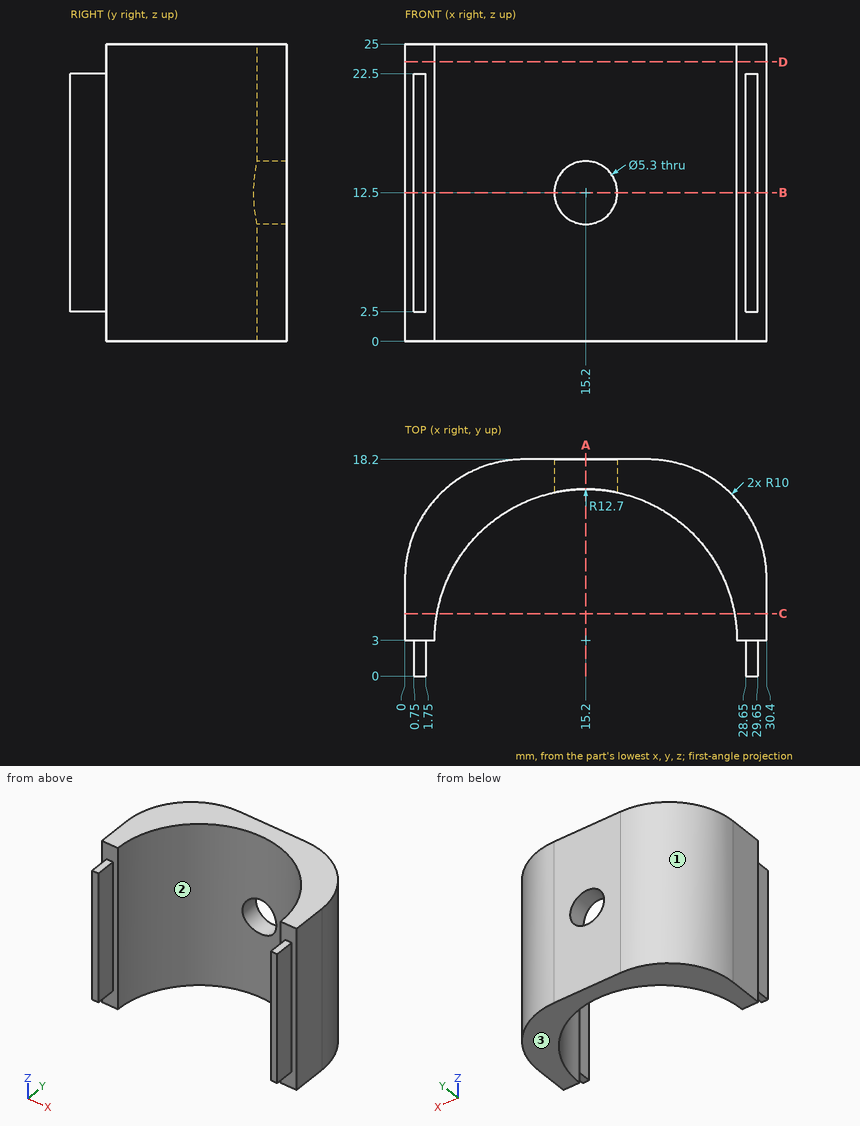
Geometry: see drawing. Coordinates: mm, zero at the bounding-box minimum. Coordinates: 2 decimals unless noted, no trailing zeros. Write each loop counter-clockwise with the first axis right and the second up, starting at its lowest first coordinate (ties: lowest second). Pieces come first, ordered by that corner, then holes. Notation, with made-up numbers: (-37, -19) - (-2, -19) arc R16 cw to (-2, -1) - close; hole circle Ø10 at (-18.5, -38.75). An arc over 180 degrees is marked (long way). Put each result on its own line as item: value. Start each with the question number.
1) Contact query for flat-ended pins moving along their axis: pin 1 (6 mm diameter, centred on x = 15.2, z = 12.5, fed in from -Y); pin 2 (3 mm diameter, centred on x = 1, z = 11.5, fed in from -Y); pin 3 (4 mm diameter, centred on y = 13, z = 18.5, fed in from +X); pin 4 (2.5 mm diameter, centred on y = 1, z = 8, fed in from -X). Output: stop coordinate, or through.
2) Cut plane B-B (z = 12.5). Return the cut outline in (x, y).
3) Ray query, L1, parallel to Z at x = 15.2, y = 16.65; L2, parallel to X at y = 2.5, z = 22; L3, parallel to X at y = 11.5, z = 10.75. Return the intervals inside material, ascending.
4) Cut plane C-C (y = 5.25). Return the cut outline in (x, z), plus the area to 3 significant figures.
5) Mould query, pull axis X, two halves, no side actions, for the marked faces 1, 2 and 3. Classes: pulls with the +X half, pulls with the -X half, needs draft (parallel to the pull), parting line crosses it, or undercut.
6) Cut plane D-D (z = 23.5). Return the cut outline in (x, y), plus the area to 3 significant figures.
7) Cut plane A-A (x = 15.2). Return the cut outline in (y, z), plus the area to 4 significant figures.
Resolved:
1. pin 1: stops at y = 15.34
1. pin 2: stops at y = 0
1. pin 3: stops at x = 30
1. pin 4: stops at x = 0.75
2. outline: (0, 3) - (0.75, 3) - (0.75, 0) - (1.75, 0) - (1.75, 3) - (2.5, 3) arc R12.7 cw to (12.55, 15.42) - (12.55, 18.2) - (10, 18.2) arc R10 ccw to (0, 8.2) - close; (17.85, 15.42) arc R12.7 cw to (27.9, 3) - (28.65, 3) - (28.65, 0) - (29.65, 0) - (29.65, 3) - (30.4, 3) - (30.4, 8.2) arc R10 ccw to (20.4, 18.2) - (17.85, 18.2) - close
3. L1: z = 0 to 9.85, 15.15 to 25
3. L2: x = 0.75 to 1.75, 28.65 to 29.65
3. L3: x = 0.56 to 5.76, 24.64 to 29.84
4. outline: (0, 0) - (2.7, 0) - (2.7, 25) - (0, 25) - close; (27.7, 0) - (30.4, 0) - (30.4, 25) - (27.7, 25) - close
4. area: 135 mm2
5. face 1: pulls with the -X half
5. face 2: undercut
5. face 3: needs draft
6. outline: (0, 3) - (2.5, 3) arc R12.7 cw to (27.9, 3) - (30.4, 3) - (30.4, 8.2) arc R10 ccw to (20.4, 18.2) - (10, 18.2) arc R10 ccw to (0, 8.2) - close
6. area: 166 mm2
7. outline: (15.7, 0) - (18.2, 0) - (18.2, 9.85) - (15.7, 9.85) - close; (15.7, 15.15) - (18.2, 15.15) - (18.2, 25) - (15.7, 25) - close
7. area: 49.25 mm2
